Check sheet for the modelled part. Datum: model origin and axes. Units: mm. A direction names the side the tool comes from. Give positions to 0.01 mm unless a question says otherwise; leave off trailing zeros. Order: outer loops, then holes, each group sorted by start corner. A loop starts at its lowest first (then second) coordinate and runs counter-clockwise, first axis right, second up. Notation, with made-up numbers: M 56,25 L 69,25 A26 ccw 69,61 Z; hole C 43.5,5.5 d9. An arc over 180 degrees is marked long. One line per question, with ' | ' between items. Start each with the question number.
```python
from build123d import *

# Parameters (mm, degrees)
F1_DEPTH = 304.8
F3_DEPTH = 37.6682579939
F5_D     = 12.7
F7_DEPTH = 38.1


with BuildPart() as f1:
    # F0 (on Right) → F1 (new body)
    with BuildSketch(Plane.YZ):
        with BuildLine():
            Line((-31.75, 37.6672579939), (-31.75, 0))
            Line((-31.75, 0), (31.75, 0))
            Line((31.75, 0), (31.75, 37.6672579939))
            Line((31.75, 37.6672579939), (12.8542501479, 37.6672579939))
            ThreePointArc((12.8542501479, 37.6672579939), (0, 25.2384677231), (-12.8542501479, 37.6672579939))
            Line((-12.8542501479, 37.6672579939), (-31.75, 37.6672579939))
        make_face()
    extrude(amount=F1_DEPTH)

    # F2 (on face) → F3 (cut, through all)
    with BuildSketch(Plane(origin=(0, 0, 0), x_dir=(1, 0, 0), z_dir=(0, 0, -1))):
        with BuildLine():
            Line((304.8, -6.5), (304.8, 6.5))
            ThreePointArc((304.8, 6.5), (298.3, 0), (304.8, -6.5))
        make_face()
    extrude(amount=-F3_DEPTH, mode=Mode.SUBTRACT)

    # F5 (through all)
    with Locations(Plane(origin=(0, 0, 0), x_dir=(1, 0, 0), z_dir=(0, 0, -1))):
        with Locations((25.4, 0), (279.4, 0)):
            Hole(F5_D / 2)

    # F6 (on face) → F7 (join)
    with BuildSketch(Plane(origin=(0, 0, 0), x_dir=(1, 0, 0), z_dir=(0, 0, -1))):
        with BuildLine():
            Line((304.8, -57.15), (304.8, -31.75))
            Line((304.8, -31.75), (279.4, -31.75))
            add(Edge.make_bspline(
                [(279.4, -31.75), (280.6196464062, -44.9519572545), (281.6562352616, -72.7591128188), (267.4659060578, -133.5460316096), (219.311230836, -155.2848931595), (196.3723528224, -160.6784621447), (192.0268553365, -161.6276637507)],
                knots=[0, 0, 0, 0, 0.2247705993, 0.4917972226, 0.7698647046, 0.837979119, 0.837979119, 0.837979119, 0.837979119], degree=3))
            ThreePointArc((192.0268553365, -161.6276637507), (190.7858628977, -166.9955827691), (185.8158122141, -169.3732314025))
            Line((185.8158122141, -169.3732314025), (185.8158122141, -182.2608020978))
            ThreePointArc((185.8158122141, -182.2608020978), (189.717508907, -183.6558096923), (191.912954164, -187.1699672577))
            add(Edge.make_bspline(
                [(206.1138840691, -183.6896836758), (201.2935156589, -184.8995347049), (196.5975482437, -186.0418094447), (191.912954164, -187.1699672577)],
                knots=[0, 0, 0, 0, 14.7614757351, 14.7614757351, 14.7614757351, 14.7614757351], degree=3))
            add(Edge.make_bspline(
                [(304.8, -57.15), (299.6183479782, -88.5960237562), (294.5771500768, -152.4240335574), (233.688003705, -172.914172303), (206.1138840691, -183.6896836758)],
                knots=[0, 0, 0, 0, 0.5045633421, 1, 1, 1, 1], degree=3))
        make_face()
        with BuildLine():
            Line((279.4, 31.75), (304.8, 31.75))
            Line((304.8, 31.75), (304.8, 57.15))
            add(Edge.make_bspline(
                [(304.8, 57.15), (299.6183479782, 88.5960237562), (294.5771500768, 152.4240335574), (233.688003705, 172.914172303), (206.1138840691, 183.6896836758)],
                knots=[0, 0, 0, 0, 0.5045633421, 1, 1, 1, 1], degree=3))
            add(Edge.make_bspline(
                [(206.1138840691, 183.6896836758), (191.930532214, 187.2495242062), (178.8241938518, 190.2243165594), (163.9156103992, 193.9758807421)],
                knots=[0, 0, 0, 0, 43.433859497, 43.433859497, 43.433859497, 43.433859497], degree=3))
            Line((163.9156103992, 193.9758807421), (163.9156103992, 168.5758807421))
            add(Edge.make_bspline(
                [(279.4, 31.75), (280.6196464062, 44.9519572545), (281.6562352616, 72.7591128188), (267.4659060578, 133.5460316096), (206.5878868967, 161.0286970804), (175.8306996904, 164.2202895611), (163.9156103992, 168.5758807421)],
                knots=[0, 0, 0, 0, 0.2247705993, 0.4917972226, 0.7698647046, 1, 1, 1, 1], degree=3))
        make_face()
    extrude(amount=-F7_DEPTH)


solid = f1.part
```
Item 1: Section check B-B, the plane y = 0. Record the cut outline in (x, z).
Item 2: Section check C-C, the plane x = 152. Record the cut outline in (y, z).
Item 3: Set-up check for faces 1 (the face through (150, 22, 37.667)), 2 (the face through (138, 31.75, 19)), 3 (the face through (163.916, -181, 19)), 4 (the face through (260, -131, 38.1)), 5 (the face through (185.816, 176, 19)): record each of +Z, -Z, +X, -X, +Y, -Y from which the full face is reachable in a straight line by a thin tool's end or side.
Item 4: Go/stop test with flat-tipped pins: P1, Ø6, axis at x = 144.5, z = 5, coming from the -Y side; P2, Ø9.5, axis at x = 145.5, y = -24, coming from the +Z side; P3, Ø14, axis at y = 174.5, z = 25.5, coming from the -X side. Record where each tip stops, or that it passes through.
Item 5: Draft check along X on faces 6 (the face through (0, 0, 19)), 7 (the face through (304.8, 32, 19)), 8 (the face through (31.744, -0.279, 13.646)), 9 (the face through (285.744, -0.279, 13.646)). Enter one of: released by +X, released by -X, zero draft, split by the parting line, or undercut.
Item 6: Section check A-A, the plane x = 25.4. Record the cut outline in (y, z), then the cut area to 3 significant figures.
Item 7: Section check D-D, the plane z = 14.5. State how many separate pieces and enclosed holes the cut face has, then the cut area to 3 significant figures.
Item 8: Scan lines: probe 1 along Y at (x, z) = (25.4, 13.5); probe 2 along Y at (x, z) = (194, 14); probe 3 along Y at (x, z) = (224, 3). Record each from-to range of solid material in increasing order. Write a range as [from, to].
Reported:
1) outline: M 0,0 L 19.05,0 L 19.05,25.24 L 0,25.24 Z; M 31.75,0 L 273.05,0 L 273.05,25.24 L 31.75,25.24 Z; M 285.75,0 L 298.3,0 L 298.3,25.24 L 285.75,25.24 Z
2) outline: M -31.75,0 L 31.75,0 L 31.75,37.67 L 12.85,37.67 A12.86 cw -12.85,37.67 L -31.75,37.67 Z
3) face 1: +Z, +X, -X | face 2: +Z, -Z, -X | face 3: +Z, -Z, -X, -Y | face 4: +Z, +X, -X, +Y, -Y | face 5: +Z, -Z, -X, +Y
4) P1: stops at y = -31.75 | P2: stops at z = 37.67 | P3: stops at x = 185.82
5) face 6: released by -X | face 7: released by +X | face 8: undercut | face 9: undercut
6) outline: M -31.75,0 L -6.35,0 L -6.35,26.92 A12.86 cw -12.85,37.67 L -31.75,37.67 Z; M 6.35,0 L 31.75,0 L 31.75,37.67 L 12.85,37.67 A12.86 cw 6.35,26.92 Z | area: 1,820 mm^2
7) separate pieces: 1 | enclosed holes: 2 | area: 29,200 mm^2
8) probe 1: y = [-31.75, -6.35], [6.35, 31.75] | probe 2: y = [-186.67, -161.19], [-31.75, 31.75], [161.19, 186.67] | probe 3: y = [-176.75, -151.82], [-31.75, 31.75], [151.82, 176.75]
